For this review, take the finished solid that the model builds, in its own axes (mm). Give positions to 0.01 mm unless a question says otherwise; leave off trailing zeros. Write each loop counter-clockwise with the first axis right and the second up, starting at its lowest first coordinate (ties: lowest second). Pieces come first, ordered by that corner, then holes. Notation, with made-up numbers: (31, 19.25) -> (44, 19.25) arc R9 ccw to (44, 25.25) -> close; hole circle Ø11 at (76, -6.75). An arc over 180 degrees is marked (long way). Answer as CSV lines item,"result".
```python
from build123d import *

# Parameters (mm, degrees)
SKETCH1_W          = 11
SKETCH1_H          = 2.9
SKETCH2_R          = 1.5
CUT_EXTRUDE1_DEPTH = 10
CHAMFER1_SIZE      = 0.5


with BuildPart() as part:
    # Sketch1 → Revolve1 (revolve)
    with BuildSketch(Plane.XY):
        with Locations((0, 3.95)):
            Rectangle(SKETCH1_W, SKETCH1_H)
    revolve(axis=Axis((0, 0, 0), (-1, 0, 0)))

    # Sketch2 → Cut-Extrude1 (cut)
    with BuildSketch(Plane(origin=(0, 0, 0), x_dir=(1, 0, 0), z_dir=(0, 1, 0))):
        with Locations((-2.75, 0)):
            Circle(SKETCH2_R)
    extrude(amount=-CUT_EXTRUDE1_DEPTH, mode=Mode.SUBTRACT)

    # Chamfer1
    chamfer1_edges = [part.edges().sort_by_distance(p)[0] for p in [
        (-5.5, -5.4, 0),
        (5.5, -5.4, 0),
        (5.5, -2.5, 0),
        (-5.5, -2.5, 0),
    ]]
    chamfer(chamfer1_edges, length=CHAMFER1_SIZE)


solid = part.part
```
Q1. Add section B-B (y = 0). Write out the cut boundary in (x, z).
Answer block:
outline,"(-5.5, -4.9) -> (-5, -5.4) -> (5, -5.4) -> (5.5, -4.9) -> (5.5, -3) -> (5, -2.5) -> (-5, -2.5) -> (-5.5, -3) -> close; (-5.5, 3) -> (-5, 2.5) -> (5, 2.5) -> (5.5, 3) -> (5.5, 4.9) -> (5, 5.4) -> (-5, 5.4) -> (-5.5, 4.9) -> close"
Q2. To check wall thickness, follow probe 1 along Z at (x, y) = (1.5, 0); probe 2 along X at (y, z) = (-3.4, 0). State the ranges of each line that lie inside material, in increasing order. Write a range as [from, to].
Answer block:
probe 1,"z = [-5.4, -2.5], [2.5, 5.4]"
probe 2,"x = [-5.5, -4.25], [-1.25, 5.5]"
Q3. Clearance check with a flat-ended pin moving along its axis: pin 1 (1.5 mm diameter, centred on x = 4, z = -1, fed in from +Y). State where the tip first meets the part, or that it passes through.
Answer block:
pin 1,"stops at y = 5.39"
Q4. Add section A-A (z = 0). Write out the cut boundary in (x, y).
Answer block:
outline,"(-5.5, -4.9) -> (-5, -5.4) -> (-4.25, -5.4) -> (-4.25, -2.5) -> (-5, -2.5) -> (-5.5, -3) -> close; (-5.5, 3) -> (-5, 2.5) -> (5, 2.5) -> (5.5, 3) -> (5.5, 4.9) -> (5, 5.4) -> (-5, 5.4) -> (-5.5, 4.9) -> close; (-1.25, -5.4) -> (5, -5.4) -> (5.5, -4.9) -> (5.5, -3) -> (5, -2.5) -> (-1.25, -2.5) -> close"
Q5. Add section C-C (x = 1.5). Write out the cut boundary in (y, z).
Answer block:
outline,"circle Ø10.8 at (0, 0); hole circle Ø5 at (0, 0)"
Q6. Draft analysis for pull direction X (two halves, no side actions). For faces 1 (the flat face through (-5.5, 0.1, 3.2)), 2 (the flat face through (5.5, 0.1, 3.2)), 3 (the cylindrical face through (-1.364, -3.676, 0.575)), state which applies: released by +X, released by -X, zero draft, split by the parting line, or undercut.
Answer block:
face 1,"released by -X"
face 2,"released by +X"
face 3,"undercut"
Q7. Add section D-D (x = -2.75). Write out the cut boundary in (y, z).
Answer block:
outline,"(-5.19, -1.5) arc R5.4 ccw (long way) to (-5.19, 1.5) -> (-2, 1.5) arc R2.5 cw (long way) to (-2, -1.5) -> close"
